Could you check a few things on this model? Use its own coordinates, in mm. A direction names the side the tool comes from. Give positions to 0.01 mm unless a question says otherwise; leave off trailing zeros. Loops run counter-clockwise (first coordinate to the right, second up) from the corner with the lowest first, then second, coordinate; pieces in that order, holes last. Notation, with made-up numbers: M 23,89 L 39,89 A18 cw 39,113 Z; hole C 7,22 d1. An arc over 180 degrees is marked long. Use a Markdown table: item, result. Add a question column.
1) If I drill on line 1 along X through (y, z) = (-1.3, 1.6); line 2 along X through (y, z) = (-0.5, 2.9); line 3 along Y through (x, z) = (2, 2.3), over which ranges is the centre line in solid material (lowest first)? Write a range as [from, to].
2) Which directions (+Z, -Z, +X, -X, +Y, -Y) give clear straight access to the entire face, cutting with the end or side of a thin tool? Please do faces 1 (the flat face through (17, -2.027, 2)), 2 (the flat face through (6.131, -1.2, -0.5)), 3 (the cylindrical face through (8.13, -1.24, 2.48)), 4 (the flat face through (3.6, -0.227, -0.5)), 5 (the flat face through (1.131, -1.2, -0.5)).
3) Suppose I cut it at C-C on z = -0.6. List the corners of the cut face in (x, y) for me, and give its area (3 significant figures).
4) Will these pins go through, and if not, where does the flat tip stop? pin 1 Ø0.5 at (y, z) = (-1, -0.5) entering from -X; pin 2 Ø2.5 at (x, z) = (18, 2) entering from -Y; pin 3 Ø0.5 at (x, z) = (4, -0.5) entering from +Y; pin 4 Ø0.8 at (y, z) = (-1.5, -0.5) entering from +X.
5) Suppose I cut it at B-B on x = 16.5. List the corners of the cut face in (y, z) for me.
6) Suppose I cut it at A-A on z = 2.95. List the corners of the cut face in (x, y) for me.
7) Suppose I cut it at D-D on y = -1.4. List the corners of the cut face in (x, z) for me, and give its area (3 significant figures).
```python
from build123d import *

# Parameters (mm, degrees)
F0_W     = 25
F0_H     = 4
F1_DEPTH = 1
F3_DEPTH = 3
F4_R     = 0.2
F5_W     = 5
F5_H     = 2
F6_DEPTH = 1


with BuildPart() as f1:
    # F0 (on Top) → F1 (new body)
    with BuildSketch(Plane.XY):
        with Locations((10.130869, -1.226871)):
            Rectangle(F0_W, F0_H)
    extrude(amount=F1_DEPTH)

    # F2 (on face) → F3 (join)
    with BuildSketch(Plane.XY.offset(1)):
        with BuildLine():
            ThreePointArc((-0.669131, -0.426871), (-1.469131, -1.226871), (-0.669131, -2.026871))
            Line((-0.669131, -2.026871), (7.330869, -2.026871))
            ThreePointArc((7.330869, -2.026871), (8.130869, -1.226871), (7.330869, -0.426871))
            Line((7.330869, -0.426871), (-0.669131, -0.426871))
        make_face()
        with BuildLine():
            ThreePointArc((12.930869, -0.426871), (12.130869, -1.226871), (12.930869, -2.026871))
            Line((12.930869, -2.026871), (20.930869, -2.026871))
            ThreePointArc((20.930869, -2.026871), (21.730869, -1.226871), (20.930869, -0.426871))
            Line((20.930869, -0.426871), (12.930869, -0.426871))
        make_face()
    extrude(amount=F3_DEPTH)

    # F4
    f4_edges = [f1.edges().sort_by_distance(p)[0] for p in [
        (22.630869, 0.773129, 0.5),
        (22.630869, -3.226871, 0.5),
        (-2.369131, -3.226871, 0.5),
        (-2.369131, 0.773129, 0.5),
    ]]
    fillet(f4_edges, radius=F4_R)

    # F5 (on face) → F6 (join)
    with BuildSketch(Plane(origin=(0, 0, 0), x_dir=(1, 0, 0), z_dir=(0, 0, -1))):
        with Locations((3.630869, 1.226871)):
            Rectangle(F5_W, F5_H)
        with Locations((16.630869, 1.226871)):
            Rectangle(F5_W, F5_H)
    extrude(amount=F6_DEPTH)


solid = f1.part
```
Answer block:
| question | item | result |
|---|---|---|
| 1 | line 1 | x = [-1.47, 8.13], [12.13, 21.73] |
| 1 | line 2 | x = [-1, 7.67], [12.6, 21.27] |
| 1 | line 3 | y = [-2.03, -0.43] |
| 2 | face 1 | +Z, +X, -X, -Y |
| 2 | face 2 | -Z, +Y, -Y |
| 2 | face 3 | +Z |
| 2 | face 4 | -Z, +X, -X, +Y |
| 2 | face 5 | -Z, -X, +Y, -Y |
| 3 | outline | M 1.13,-2.23 L 6.13,-2.23 L 6.13,-0.23 L 1.13,-0.23 Z; M 14.13,-2.23 L 19.13,-2.23 L 19.13,-0.23 L 14.13,-0.23 Z |
| 3 | area | 20.0 mm^2 |
| 4 | pin 1 | stops at x = 1.13 |
| 4 | pin 2 | stops at y = -3.23 |
| 4 | pin 3 | stops at y = -0.23 |
| 4 | pin 4 | stops at x = 19.13 |
| 5 | outline | M -3.23,0 L -2.23,0 L -2.23,-1 L -0.23,-1 L -0.23,0 L 0.77,0 L 0.77,1 L -0.43,1 L -0.43,4 L -2.03,4 L -2.03,1 L -3.23,1 Z |
| 6 | outline | M -0.67,-2.03 L 7.33,-2.03 A0.8 ccw 7.33,-0.43 L -0.67,-0.43 A0.8 ccw Z; M 12.93,-2.03 L 20.93,-2.03 A0.8 ccw 20.93,-0.43 L 12.93,-0.43 A0.8 ccw Z |
| 7 | outline | M -2.37,0 L 1.13,0 L 1.13,-1 L 6.13,-1 L 6.13,0 L 14.13,0 L 14.13,-1 L 19.13,-1 L 19.13,0 L 22.63,0 L 22.63,1 L 21.71,1 L 21.71,4 L 12.15,4 L 12.15,1 L 8.11,1 L 8.11,4 L -1.45,4 L -1.45,1 L -2.37,1 Z |
| 7 | area | 92.4 mm^2 |
